The model under review builds one solid part; all positions refer to its coordinate system, in mm. Face numbers are marked on the shaded views. A direction names the side the tool comes from. Round coordinates to 2 decimals unless told otherwise and drop trailing zeros. Order: outer loops, then holes, each group sorted by start corner. A loop starts at its lowest first (then second) coordinate and runs counter-clockwise, first axis right, second up.
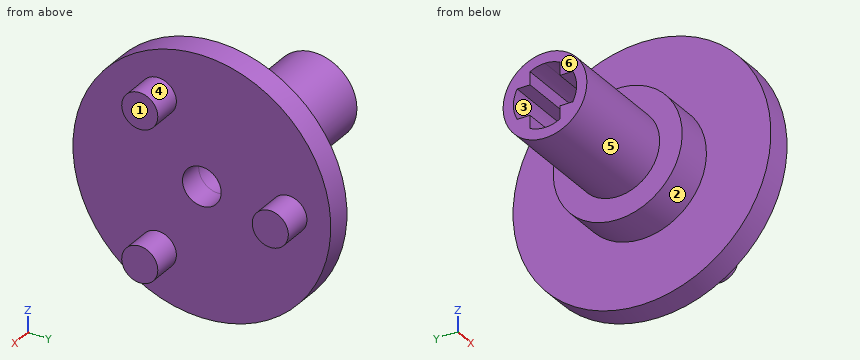
from build123d import *

# Parameters (mm, degrees)
SKETCH_1_R          = 1.4
EXTRUDE_1_DEPTH     = 2.3
EXTRUDE_1_2_DEPTH   = 2.3
EXTRUDE_1_3_DEPTH   = 2.3
SKETCH_2_R          = 10
SKETCH_2_R_2        = 1.5
EXTRUDE_2_DEPTH     = 2
SKETCH_3_R          = 5
SKETCH_3_R_2        = 1.5
EXTRUDE_3_DEPTH     = 4
SKETCH_4_R          = 3.25
SKETCH_4_R_2        = 2.45
EXTRUDE_4_DEPTH     = 8
EXTRUDE_5_DEPTH     = 8
CUT_EXTRUDE_START   = -1
SKETCH_4_6_R        = 5
SKETCH_4_6_R_2      = 3.25
CUT_EXTRUDE_1_DEPTH = 1


with BuildPart() as part:
    # Sketch 1 → Extrude 1 (new body)
    with BuildSketch(Plane(origin=(0, 0, 0), x_dir=(0, 0, -1), z_dir=(1, 0, 0))):
        with Locations((0, 6.75)):
            Circle(SKETCH_1_R)
    extrude(amount=EXTRUDE_1_DEPTH)



with BuildPart() as body_2:
    # Sketch 1 → Extrude 1 2 (new body)
    with BuildSketch(Plane(origin=(0, 0, 0), x_dir=(0, 0, -1), z_dir=(1, 0, 0))):
        with Locations((5.845671476, -3.375)):
            Circle(SKETCH_1_R)
    extrude(amount=EXTRUDE_1_2_DEPTH)


with BuildPart() as body_3:
    # Sketch 1 → Extrude 1 3 (new body)
    with BuildSketch(Plane(origin=(0, 0, 0), x_dir=(0, 0, -1), z_dir=(1, 0, 0))):
        with Locations((-5.845671476, -3.375)):
            Circle(SKETCH_1_R)
    extrude(amount=EXTRUDE_1_3_DEPTH)


with BuildPart() as part_1:
    add(part.part)

    add(body_2.part)  # Extrude 2 merges body 2

    add(body_3.part)  # Extrude 2 merges body 3
    # Sketch 2 → Extrude 2 (add)
    with BuildSketch(Plane(origin=(0, 0, 0), x_dir=(0, 0, -1), z_dir=(1, 0, 0))):
        Circle(SKETCH_2_R)
        Circle(SKETCH_2_R_2, mode=Mode.SUBTRACT)
    extrude(amount=-EXTRUDE_2_DEPTH)

    # Sketch 3 → Extrude 3 (add)
    with BuildSketch(Plane.ZY.offset(2)):
        with Locations(Location((0, 0, 0), (0, 0, 180))):
            Circle(SKETCH_3_R)
        with Locations(Location((0, 0, 0), (0, 0, 180))):
            Circle(SKETCH_3_R_2, mode=Mode.SUBTRACT)
    extrude(amount=EXTRUDE_3_DEPTH)

    # Sketch 4 → Extrude 4 (add)
    with BuildSketch(Plane.ZY.offset(6)):
        Circle(SKETCH_4_R)
        Circle(SKETCH_4_R_2, mode=Mode.SUBTRACT)
    extrude(amount=EXTRUDE_4_DEPTH)

    # Sketch 4_3 → Extrude 5 (add)
    with BuildSketch(Plane.ZY.offset(6)):
        with BuildLine():
            Line((2.158689242, -1.158689242), (1.158689242, -1.158689242))
            Line((1.158689242, -1.158689242), (1.158689242, -2.158689242))
            ThreePointArc((1.158689242, -2.158689242), (1.732411614, -1.732411614), (2.158689242, -1.158689242))
        make_face()
        with BuildLine():
            ThreePointArc((2.158689242, 1.158689242), (1.732411614, 1.732411614), (1.158689242, 2.158689242))
            Line((1.158689242, 2.158689242), (1.158689242, 1.158689242))
            Line((1.158689242, 1.158689242), (2.158689242, 1.158689242))
        make_face()
        with BuildLine():
            Line((-1.158689242, 1.158689242), (-1.158689242, 2.158689242))
            ThreePointArc((-1.158689242, 2.158689242), (-1.732411614, 1.732411614), (-2.158689242, 1.158689242))
            Line((-2.158689242, 1.158689242), (-1.158689242, 1.158689242))
        make_face()
        with BuildLine():
            Line((-1.158689242, -2.158689242), (-1.158689242, -1.158689242))
            Line((-1.158689242, -1.158689242), (-2.158689242, -1.158689242))
            ThreePointArc((-2.158689242, -1.158689242), (-1.732411614, -1.732411614), (-1.158689242, -2.158689242))
        make_face()
    extrude(amount=EXTRUDE_5_DEPTH)

    # Sketch 4_6 → Cut-Extrude 1 (cut)
    with BuildSketch(Plane.ZY.offset(6).offset(CUT_EXTRUDE_START)):
        with Locations(Location((0, 0, 0), (0, 0, 180))):
            Circle(SKETCH_4_6_R)
        Circle(SKETCH_4_6_R_2, mode=Mode.SUBTRACT)
    extrude(amount=CUT_EXTRUDE_1_DEPTH, mode=Mode.SUBTRACT)


solid = part_1.part
(1) We need section C-C (y = 7.25). Give the boundary of the cut face in (x, z).
(2) Clearance check with flat-ended pins moving along their axes: P1, Ø1.5, axis at x = -0.5, z = -3, coming from the +Y side; P2, Ø3, axis at x = -2, z = 2, coming from the +Y side; P3, Ø1.1, axis at x = -10.5, y = -1.5, coming from the -Z side. State where each tip first meets the part, or that it passes through.
(3) Tool access review of the marked faces 4, 5 and 6: name each direction out of +Z, -Z, +X, -X, +Y, -Y from which nothing blocks a thin tool from reaching the whole face with its end or side.
(4) To check wall thickness, follow L1, parallel to Y at x = -1.5, z = 0; L2, parallel to Y at x = -8.25, z = 0; L3, parallel to X at y = 5.5, z = 8.25. State the ranges of each line that lie inside material, in increasing order.
(5) We need section A-A (z = 0). Give the boundary of the cut face in (x, y), and give its area (3 significant figures).
(6) We need section D-D (z = -8). Give the boundary of the cut face in (x, y), and give its area (3 significant figures).
(7) We need section B-B (x = -10.75). Give the boundary of the cut face in (y, z).
(8) The part is to be moulded in two halves that separate along Y. For the marked faces 1, 2 and 3, say which applies: pulls with the +Y half, pulls with the -Y half, needs draft (parallel to the pull), parting line crosses it, or undercut.
Verdict:
1. outline: (-2, -6.89) - (0, -6.89) - (0, -1.31) - (2.3, -1.31) - (2.3, 1.31) - (0, 1.31) - (0, 6.89) - (-2, 6.89) - close
2. P1: stops at y = 9.74
2. P2: stops at y = 9.99
2. P3: stops at z = -3.11
3. face 4: +X
3. face 5: -X
3. face 6: +Z, -Z, -X, +Y, -Y
4. L1: y = -10 to -1.5, 1.5 to 10
4. L2: y = -3.25 to -2.45, 2.45 to 3.25
4. L3: x = -2 to 0
5. outline: (-14, -3.25) - (-5, -3.25) - (-5, -5) - (-2, -5) - (-2, -10) - (0, -10) - (0, -1.5) - (-6, -1.5) - (-6, -2.45) - (-14, -2.45) - close; (-14, 2.45) - (-6, 2.45) - (-6, 1.5) - (0, 1.5) - (0, 5.35) - (2.3, 5.35) - (2.3, 8.15) - (0, 8.15) - (0, 10) - (-2, 10) - (-2, 5) - (-5, 5) - (-5, 3.25) - (-14, 3.25) - close
5. area: 77.7 mm2
6. outline: (-2, -6) - (0, -6) - (0, 6) - (-2, 6) - close
6. area: 24.0 mm2
7. outline: circle Ø6.5 at (0, 0); hole (-2.16, -1.16) - (-1.16, -1.16) - (-1.16, -2.16) arc R2.45 ccw to (1.16, -2.16) - (1.16, -1.16) - (2.16, -1.16) arc R2.45 ccw to (2.16, 1.16) - (1.16, 1.16) - (1.16, 2.16) arc R2.45 ccw to (-1.16, 2.16) - (-1.16, 1.16) - (-2.16, 1.16) arc R2.45 ccw to start
8. face 1: needs draft
8. face 2: parting line crosses it
8. face 3: undercut
